Check sheet for the modelled part. Datum: model origin and axes. Units: mm. A direction names the side the tool comes from. Round coordinates to 2 decimals unless told otherwise and drop trailing zeros. Loops run counter-clockwise (first coordinate to the right, second up) from the corner with the lowest first, then second, coordinate; pieces in that order, holes last. Notation, with made-up numbers: (54.25, -37.75) -> (108.25, -37.75) arc R17 ccw to (108.25, -9.75) -> close; hole circle Ø8 at (-33.75, 47.25). An arc over 180 degrees is marked (long way). One line per item, written item: value. Start each with the question number.
1. Cross-section at D-D on z = 55. Record the cut outline in (x, y).
2. Set-up check for faces 1 (the face through (-5.9, -15.86, 36.9)), 2 (the face through (-62.778, -12.535, 19.708)), 3 (the face through (-8, -88, 20)): record each of +Z, -Z, +X, -X, +Y, -Y from which the full face is reachable in a straight line by a thin tool's end or side.
3. Release check for a two-part mould opening along Z. For faces 4 (the face through (-23.3, -12.46, 34.63)), 5 (the face through (-35.11, -15.86, 5.9)), 6 (the face through (-7.5, -85, 14.5)) record: +Z half, -Z half, draft (parallel to the pull), parting line (faces both ways), or undercut.
4. Cross-section at B-B on z = 11. Record the cut outline in (x, y).
5. Go/stop test with flat-tipped pins: pin 1 (8 mm diameter, centred on x = -20.98, z = 36.76, fed in from +Y); pin 2 (16.5 mm diameter, centred on x = -48.5, z = 45.5, fed in from -Y); pin 3 (8 mm diameter, centred on x = -26.5, y = -33.5, fed in from +Z). Record where each tip stops, or that it passes through.
6. Cross-section at C-C on y = -57. Record the cut outline in (x, z), then the cut area to 3 significant figures.
7. Cross-section at A-A on x = -15. Record the cut outline in (y, z), then the cut area to 3 significant figures.
8. Material ranges on L1, parallel to X at y = -13, z = 15; L2, parallel to Z at x = -15, y = -12.55; L3, parallel to X at y = -65.5, z = 26, recorded low to high.
from build123d import *

# Parameters (mm, degrees)
SALIENTE_EXTRUIR1_DEPTH = 5
CROQUIS2_W              = 5
CROQUIS2_H              = 90
SALIENTE_EXTRUIR2_DEPTH = 60
CORTAR_EXTRUIR1_DEPTH   = 5
SALIENTE_EXTRUIR3_DEPTH = 5
REDONDEO1_R             = 3
CROQUIS5_W              = 58
CROQUIS5_H              = 5
SALIENTE_EXTRUIR4_DEPTH = 60
CORTAR_EXTRUIR2_DEPTH   = 5
REDONDEO2_R             = 3
REDONDEO3_R             = 3
CROQUIS7_R              = 1.75
CROQUIS7_R_2            = 3.15
CORTAR_EXTRUIR3_DEPTH   = 5


with BuildPart() as part:
    # Croquis1 → Saliente-Extruir1 (new body)
    with BuildSketch(Plane.XY):
        with BuildLine():
            Line((-63, 0), (0, 0))
            Line((0, 0), (0, -90))
            Line((0, -90), (-33, -90))
            Line((-33, -90), (-33, -48))
            ThreePointArc((-33, -48), (-41.786797, -26.786797), (-63, -18))
            Line((-63, -18), (-63, 0))
        make_face()
    extrude(amount=SALIENTE_EXTRUIR1_DEPTH)

    # Croquis2 → Saliente-Extruir2 (add)
    with BuildSketch(Plane.XY.offset(5)):
        with Locations((-2.5, -45)):
            Rectangle(CROQUIS2_W, CROQUIS2_H)
    extrude(amount=SALIENTE_EXTRUIR2_DEPTH)

    # Croquis3 → Cortar-Extruir1 (cut)
    with BuildSketch(Plane(origin=(0, 0, 0), x_dir=(0, 0, -1), z_dir=(1, 0, 0))):
        with BuildLine():
            Line((-65, -90), (-35, -90))
            Line((-35, -90), (-35, -48))
            ThreePointArc((-35, -48), (-43.786797, -26.786797), (-65, -18))
            Line((-65, -18), (-65, -90))
        make_face()
    extrude(amount=-CORTAR_EXTRUIR1_DEPTH, mode=Mode.SUBTRACT)

    # Croquis4 → Saliente-Extruir3 (add)
    with BuildSketch(Plane.XZ.offset(90)):
        Polygon((-33, 8), (-8, 8), (-8, 35), (-5, 35), (-5, 5), (-33, 5), align=None)
    extrude(amount=-SALIENTE_EXTRUIR3_DEPTH)

    # Redondeo1
    redondeo1_edges = [part.edges().sort_by_distance(p)[0] for p in [
        (-33, -87.5, 8),
        (-8, -87.5, 35),
    ]]
    fillet(redondeo1_edges, radius=REDONDEO1_R)

    # Croquis5 → Saliente-Extruir4 (add)
    with BuildSketch(Plane.XY.offset(5)):
        with Locations((-34, -12.5)):
            Rectangle(CROQUIS5_W, CROQUIS5_H)
    extrude(amount=SALIENTE_EXTRUIR4_DEPTH)

    # Croquis6 → Cortar-Extruir2 (cut)
    with BuildSketch(Plane(origin=(0, -10, 0), x_dir=(1, 0, 0), z_dir=(0, 1, 0))):
        Polygon((-63, -19.817641), (-17.817641, -65), (-63, -65), align=None)
    extrude(amount=-CORTAR_EXTRUIR2_DEPTH, mode=Mode.SUBTRACT)

    # Redondeo2
    redondeo2_edges = [part.edges().sort_by_distance(p)[0] for p in [
        (-63, -12.5, 19.817641),
        (-17.817641, -12.5, 65),
    ]]
    fillet(redondeo2_edges, radius=REDONDEO2_R)

    # Redondeo3
    redondeo3_edges = [part.edges().sort_by_distance(p)[0] for p in [
        (-34, -15, 5),
        (-5, -15, 35),
        (-5, -50, 5),
    ]]
    fillet(redondeo3_edges, radius=REDONDEO3_R)

    # Croquis7 → Cortar-Extruir3 (cut)
    with BuildSketch(Plane(origin=(0, -10, 0), x_dir=(1, 0, 0), z_dir=(0, 1, 0))):
        with Locations((-15, -55)):
            Circle(CROQUIS7_R)
        with Locations((-15, -15)):
            Circle(CROQUIS7_R)
        with Locations((-55, -15)):
            Circle(CROQUIS7_R)
        with Locations((-58.699976, -11)):
            Circle(CROQUIS7_R_2)
        with Locations((-20.975, -36.755655)):
            Circle(CROQUIS7_R_2)
    extrude(amount=-CORTAR_EXTRUIR3_DEPTH, mode=Mode.SUBTRACT)


solid = part.part
Taken from the geometry:
1. outline: (-27.82, -15) -> (-16.75, -15) -> (-16.75, -10) -> (-27.82, -10) -> close; (-13.25, -15) -> (-8, -15) arc R3 cw to (-5, -18) -> (-5, -19.72) -> (0, -19.72) -> (0, 0) -> (-5, 0) -> (-5, -10) -> (-13.25, -10) -> close
2. face 1: +Z, -X
2. face 2: +Z, -X, +Y, -Y
2. face 3: +Z, -X, -Y
3. face 4: undercut
3. face 5: +Z half
3. face 6: draft
4. outline: (-63, -15) -> (-61.85, -15) -> (-61.85, -10) -> (-63, -10) -> close; (-55.55, -15) -> (-8, -15) arc R3 cw to (-5, -18) -> (-5, -85) -> (-8, -85) -> (-8, -90) -> (0, -90) -> (0, 0) -> (-5, 0) -> (-5, -10) -> (-55.55, -10) -> close
5. pin 1: stops at y = -10
5. pin 2: stops at y = -15
5. pin 3: stops at z = 5
6. outline: (-33, 0) -> (0, 0) -> (0, 35) -> (-5, 35) -> (-5, 8) arc R3 cw to (-8, 5) -> (-33, 5) -> close
6. area: 317 mm2
7. outline: (-90, 0) -> (0, 0) -> (0, 5) -> (-10, 5) -> (-10, 13.25) -> (-15, 13.25) -> (-15, 8) arc R3 cw to (-18, 5) -> (-85, 5) -> (-85, 8) -> (-90, 8) -> close; (-15, 16.75) -> (-10, 16.75) -> (-10, 53.25) -> (-15, 53.25) -> close; (-15, 56.75) -> (-10, 56.75) -> (-10, 65) -> (-15, 65) -> close
7. area: 732 mm2
8. L1: x = -63 to -56.75, -53.25 to -16.75, -13.25 to 0
8. L2: z = 0 to 13.25, 16.75 to 53.25, 56.75 to 65
8. L3: x = -5 to 0
